For this review, take the finished solid that the model builds, in its own axes (mm). A direction names the side the tool comes from. Coordinates: 2 decimals unless noted, no trailing zeros. Loops run counter-clockwise (first coordinate to the right, second up) from the corner with the lowest first, then second, coordinate; pieces in that order, holes last. Notation, with made-up numbers: (-6.5, 54.25) -> (52.5, 54.25) arc R22 ccw to (52.5, 69.25) -> close; hole circle Ø3 at (59, 83.25). An arc over 180 degrees is marked (long way). Use a Markdown table: item, result.
from build123d import *

# Parameters (mm, degrees)
OUTLINE_DEPTH        = 40
OUTLINE_DEPTH_BACK   = 40
SKETCH1_W            = 18.25
SKETCH1_H            = 40
SKETCH2_W            = 40
SKETCH2_H            = 80
EXTRUSION15_DEPTH    = 6
CAMERA_MOUNT_D       = 24.5364
SKETCH5_R            = 17.5
SKETCH5_R_2          = 12.268
EXTRUSION19_DEPTH    = 5.9562
CUT_EXTRUDE1_START   = -3
SKETCH10_W           = 80
SKETCH10_H           = 80
SKETCH10_R           = 17.5
CUT_EXTRUDE1_DEPTH   = 3
SKETCH7_W            = 50
SKETCH7_H            = 50
EXTRUSION22_DEPTH    = 9
FILLET4_R            = 3.175
HOLE7_D              = 3.3
HOLE7_DEPTH          = 12
HOLE7_TIP            = 0.991420021
SKETCH11_OUTSIDE_W   = 105.14
SKETCH11_OUTSIDE_H   = 105.14
SKETCH11_OUTSIDE_W_2 = 74
SKETCH11_OUTSIDE_H_2 = 74
CUT_EXTRUDE2_DEPTH   = 59.588074725
CUT_EXTRUDE3_START   = -3
CUT_EXTRUDE3_DEPTH   = 3


with BuildPart() as part:
    # Sketch1 → Outline (new, two sides: drawn at the far end of the back side and taken through both)
    with BuildSketch(Plane.YZ.offset(-OUTLINE_DEPTH_BACK)):
        Polygon((18.25, 40), (5.33, 40), (0, 40), (0, 0), (18.25, 0), align=None)
        with Locations((9.125, -20)):
            Rectangle(SKETCH1_W, SKETCH1_H)
    extrude(amount=OUTLINE_DEPTH + OUTLINE_DEPTH_BACK)

    # Sketch2 → Extrusion15 (cut)
    with BuildSketch(Plane.XZ):
        Rectangle(SKETCH2_W, SKETCH2_H)
    extrude(amount=-EXTRUSION15_DEPTH, mode=Mode.SUBTRACT)

    # Camera mount (through all)
    with Locations(Plane(origin=(0, 18.25, 0), x_dir=(1, 0, 0), z_dir=(0, 1, 0))):
        with Locations((0, 0)):
            Hole(CAMERA_MOUNT_D / 2)

    # Sketch5 → Extrusion19 (add)
    with BuildSketch(Plane(origin=(0, 18.25, 0), x_dir=(-1, 0, 0), z_dir=(0, 1, 0))):
        with Locations(Location((0, 0, 0), (0, 0, 90))):
            Circle(SKETCH5_R)
        with Locations(Location((0, 0, 0), (0, 0, 90))):
            Circle(SKETCH5_R_2, mode=Mode.SUBTRACT)
    extrude(amount=EXTRUSION19_DEPTH)

    # Sketch10 → Cut-Extrude1 (cut)
    with BuildSketch(Plane(origin=(0, 18.25, 0), x_dir=(1, 0, 0), z_dir=(0, 1, 0)).offset(CUT_EXTRUDE1_START)):
        Rectangle(SKETCH10_W, SKETCH10_H)
        with Locations(Location((0, 0, 0), (0, 0, 270))):
            Circle(SKETCH10_R, mode=Mode.SUBTRACT)
    extrude(amount=CUT_EXTRUDE1_DEPTH, mode=Mode.SUBTRACT)

    # Sketch7 → Extrusion22 (cut)
    with BuildSketch(Plane.XZ):
        Rectangle(SKETCH7_W, SKETCH7_H)
    extrude(amount=-EXTRUSION22_DEPTH, mode=Mode.SUBTRACT)

    # Fillet4
    fillet4_edges = [part.edges().sort_by_distance(p)[0] for p in [
        (0, 15.25, -17.5),
        (-25, 4.5, 25),
        (25, 4.5, -25),
        (-25, 4.5, -25),
        (25, 4.5, 25),
    ]]
    fillet(fillet4_edges, radius=FILLET4_R)

    # Hole7
    with Locations(Plane(origin=(0, 0, 0), x_dir=(-1, 0, 0), z_dir=(0, -1, 0))):
        with Locations((30, 27.5), (-30, 27.5), (-30, -27.5), (30, -27.5)):
            Hole(HOLE7_D / 2, depth=HOLE7_DEPTH)
            with Locations((0, 0, -(HOLE7_DEPTH + HOLE7_TIP / 2))):  # 118° drill point
                Cone(0, HOLE7_D / 2, HOLE7_TIP, mode=Mode.SUBTRACT)

    # Sketch11 outside → Cut-Extrude2 (cut, through all)
    with BuildSketch(Plane(origin=(0, 15.25, 0), x_dir=(1, 0, 0), z_dir=(0, 1, 0))):
        Rectangle(SKETCH11_OUTSIDE_W, SKETCH11_OUTSIDE_H)
        Rectangle(SKETCH11_OUTSIDE_W_2, SKETCH11_OUTSIDE_H_2, mode=Mode.SUBTRACT)
    extrude(amount=-CUT_EXTRUDE2_DEPTH, mode=Mode.SUBTRACT)

    # Sketch13 → Cut-Extrude3 (cut)
    with BuildSketch(Plane.XZ.offset(-9).offset(CUT_EXTRUDE3_START)):
        with BuildLine():
            Line((21.825, 25), (-21.825, 25))
            ThreePointArc((-21.825, 25), (-24.07006403, 24.07006403), (-25, 21.825))
            Line((-25, 21.825), (-25, -21.825))
            ThreePointArc((-25, -21.825), (-24.07006403, -24.07006403), (-21.825, -25))
            Line((-21.825, -25), (21.825, -25))
            ThreePointArc((21.825, -25), (24.07006403, -24.07006403), (25, -21.825))
            Line((25, -21.825), (25, 21.825))
            ThreePointArc((25, 21.825), (24.07006403, 24.07006403), (21.825, 25))
        make_face()
    extrude(amount=CUT_EXTRUDE3_DEPTH, mode=Mode.SUBTRACT)


solid = part.part
(1) Mouldability with a two-part tool opening along X and no side actions: class faces 6 (the face through (-25, 6, 0)), 7 (the face through (37, 8, 1)), 8 (the face through (-4, 24.206, -12)) as pulls with the +X half, pulls with the -X half, needs draft (parallel to the pull), parting line crosses it, or undercut.
Found:
| item | result |
|---|---|
| face 6 | undercut |
| face 7 | pulls with the +X half |
| face 8 | needs draft |
(2) For pin 1 Ø5.5 at (x, z) = (30, 27.5) entering from +Y; pin 2 Ø5 at (x, z) = (8.5, 4.5) entering from +Y; pin 3 Ø2 at (x, z) = (-21.5, -23) entering from -Y; pin 4 Ø9.5 at (x, z) = (-3, -28) entering from -Y, all flat-tipped, find the tip position at first contact; note any pin that passes through.
Found:
| item | result |
|---|---|
| pin 1 | stops at y = 15.25 |
| pin 2 | passes through |
| pin 3 | stops at y = 12 |
| pin 4 | stops at y = 6 |
(3) For faces 1 (the face through (-30.215, 6.084, -29.136)), 2 (the face through (0, 6, -31)), 3 (the face through (-11.7, 15.08, -3.69)), 4 (the face through (-17, 15.25, -17)), 5 (the face through (-1, 9, 37)), list the 3-axis set-ups (+Z, -Z, +X, -X, +Y, -Y) from which the entire face can be reached by the end or side of a thin tool; tool diameter is ignored.
Found:
| item | result |
|---|---|
| face 1 | -Y |
| face 2 | +Z, -Z, -Y |
| face 3 | +Y, -Y |
| face 4 | +Y |
| face 5 | +Z, +X, -X, +Y, -Y |
(4) Take a section at A-A on y = 4.25. Write out the cut boundary in (x, z) (3 decimals), plus the area to 3 significant figures.
Found:
| item | result |
|---|---|
| outline | (-37, -37) -> (-20, -37) -> (-20, -25) -> (-21.825, -25) arc R3.175 cw to (-25, -21.825) -> (-25, 21.825) arc R3.175 cw to (-21.825, 25) -> (-20, 25) -> (-20, 37) -> (-37, 37) -> close; (20, -37) -> (37, -37) -> (37, 37) -> (20, 37) -> (20, 25) -> (21.825, 25) arc R3.175 cw to (25, 21.825) -> (25, -21.825) arc R3.175 cw to (21.825, -25) -> (20, -25) -> close; hole circle Ø3.3 at (-30, -27.5); hole circle Ø3.3 at (-30, 27.5); hole circle Ø3.3 at (30, -27.5); hole circle Ø3.3 at (30, 27.5) |
| area | 1,990 mm^2 |
(5) Take a section at D-D on x = -27. Write out the cut boundary in (y, z).
Found:
| item | result |
|---|---|
| outline | (0, -37) -> (15.25, -37) -> (15.25, 37) -> (0, 37) -> close |
(6) For line 1 along Z through (x, y) = (30, 9); line 2 along X through (y, z) = (7.75, -27.5); line 3 along Z through (x, y) = (22, 1.75), list the stretches that pass through material, from the lowest coordinate up.
Found:
| item | result |
|---|---|
| line 1 | z = -37 to -29.15, -25.85 to 25.85, 29.15 to 37 |
| line 2 | x = -37 to -31.65, -28.35 to 28.35, 31.65 to 37 |
| line 3 | z = -37 to -25, 25 to 37 |
(7) Take a section at C-C on y = 16.25. Write out the cut boundary in (x, z).
Found:
| item | result |
|---|---|
| outline | circle Ø36.72 at (0, 0); hole circle Ø24.54 at (0, 0) |
